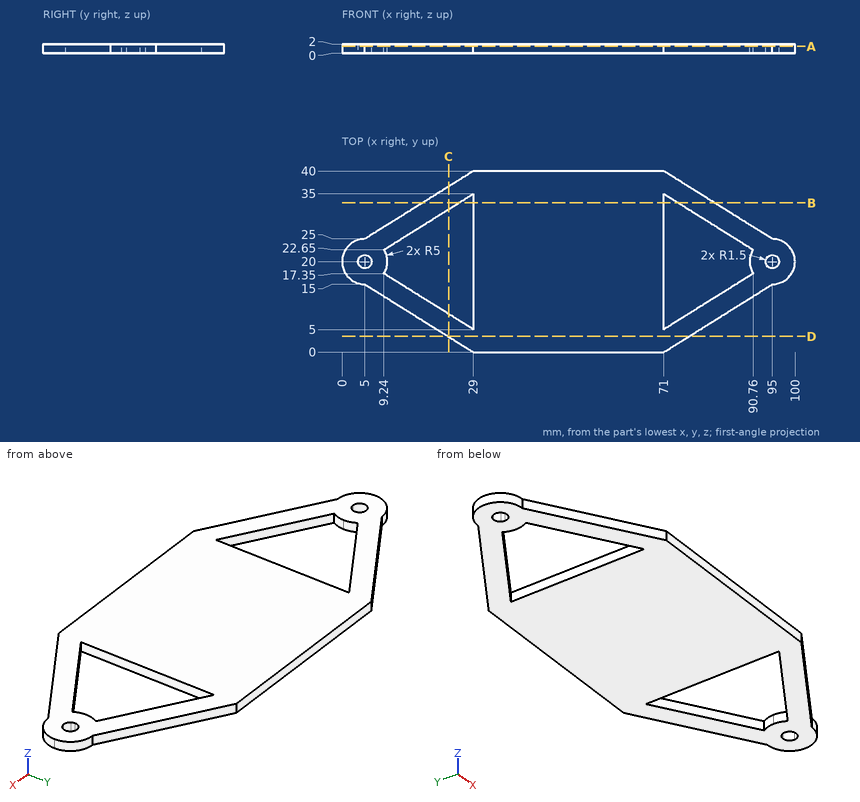
Could you check a few things on this drawing? It's one solid part, dimensions in mm from its lowest x, y, z. Give positions to 0.01 mm unless a question says otherwise; leave off trailing zeros. Order: outer loops, then holes, each group sorted by start corner. A loop starts at its lowest first (then second) coordinate and runs counter-clockwise, first axis right, second up. Notation, with made-up numbers: M 24,89.5 L 43,89.5 A23 ccw 43,125.5 Z; hole C 51.5,14.25 d5. An arc over 180 degrees is marked long. Use one line per item in the form item = value.
Item 1: If we section it at D-D, the plane y = 3.5: Write out the boundary of the cut face in (x, z), and give its area (3 significant figures).
Values follow:
outline = M 23.4,0 L 76.6,0 L 76.6,2 L 23.4,2 Z
area = 106 mm^2
Item 2: If we section it at B-B, the plane y = 33: Write out the boundary of the cut face in (x, z), and give its area (3 significant figures).
Values follow:
outline = M 17.8,0 L 25.8,0 L 25.8,2 L 17.8,2 Z; M 29,0 L 71,0 L 71,2 L 29,2 Z; M 74.2,0 L 82.2,0 L 82.2,2 L 74.2,2 Z
area = 116 mm^2
Item 3: Will these pins go through, and if not, where does the flat tip stop? pin 1 Ø0.6 at (y, z) = (18, 1) entering from +X; pin 2 Ø0.6 at (y, z) = (24, 1) entering from -X; pin 3 Ø1 at (y, z) = (8, 0.5) entering from -X.
Values follow:
pin_1 = 99.7
pin_2 = 1.64
pin_3 = 15.4
Item 4: If I drill on line 1 along X through (y, z) = (14, 1.1); line 2 along X through (y, z) = (12, 0.8); line 3 along X through (y, z) = (20.5, 0.7), over which ranges is the centre line in solid material (lowest first)? Write a range as [from, to].
Values follow:
line_1 = [6.6, 14.6], [29, 71], [85.4, 93.4]
line_2 = [9.8, 17.8], [29, 71], [82.2, 90.2]
line_3 = [0.03, 3.59], [6.41, 9.97], [29, 71], [90.03, 93.59], [96.41, 99.97]
Item 5: If we section it at C-C, the plane x = 23.5: Write out the boundary of the cut face in (y, z).
Values follow:
outline = M 3.44,0 L 8.44,0 L 8.44,2 L 3.44,2 Z; M 31.56,0 L 36.56,0 L 36.56,2 L 31.56,2 Z
Item 6: If we section it at A-A, the plane z = 1.45: Write out the boundary of the cut face in (x, y) (3 decimals), and give its area (3 significant figures).
Values follow:
outline = M 5,15 L 29,0 L 71,0 L 95,15 A5 ccw 95,25 L 71,40 L 29,40 L 5,25 A5 ccw Z; hole C 5,20 d3; hole M 9.24,17.35 L 29,5 L 29,35 L 9.24,22.65 A5 cw Z; hole M 71,5 L 90.76,17.35 A5 cw 90.76,22.65 L 71,35 Z; hole C 95,20 d3
area = 2,250 mm^2
